The listing builds one solid part. Answer for the finished solid, in the listing's coordinates (mm). A direction names the side the tool comes from. Give positions to 0.01 mm unless a question says otherwise; leave off trailing zeros. Order: outer loops, then holes, each group sorted by start corner. A loop starts at its lowest first (then second) coordinate and runs counter-clockwise, first axis right, second up. Notation, with made-up numbers: (12.25, -39) - (62.25, -39) arc R19 cw to (62.25, -24) - close; hole circle Ø4 at (52, 39). An arc over 180 degrees is marked (long way). Write each question's results on one line, items separated by ' | '. Start each with the question number.
1. Find the intervals of material crossed by L1, parallel to X at y = -3.5, z = 14; L2, parallel to Z at x = 20, y = -3.25; L3, parallel to Y at x = 9, z = 0.5, in increasing order.
2. Section B-B (x = 31.5) is taken. Give the vertices of the cut face in (y, z), and give its area (3 significant figures).
3. Section C-C (z = -6.5) is taken. Give the vertices of the cut face in (x, y), and give its area (3 significant figures).
4. Section A-A (y = -3.75) is taken. Give the vertices of the cut face in (x, z).
5. A flat-ended cylindrical pin translates along its axis: pin 1 (15 mm diameter, centred on x = -17, z = 5, fed in from -Y). Find the tip coordinate at first contact, or state that the pin passes through.
6. Which of the six approach directions +Z, -Z, +X, -X, +Y, -Y give full straight-line access (tool end or side, diameter ignored) to faces 1 (the face through (53.85, -4, 0)), 2 (the face through (-1, 0, 0))?
7. Determine the mould class of faces 3 (the face through (-1, -3, -27.06)), 4 (the face through (-4.98, -4, 0)), 5 (the face through (-5, -6.65, 22)) for opening direction Z: released by +Z, released by -Z, zero draft, split by the parting line, or undercut.
from build123d import *

# Parameters (mm, degrees)
F0_W     = 121.7
F0_H     = 54.12
F1_DEPTH = 6.65
F2_W     = 27.26
F2_H     = 40.12
F2_W_2   = 18.61
F3_DEPTH = 4.85


with BuildPart() as f1:
    # F0 (on Front) → F1 (new body)
    with BuildSketch(Plane.XZ):
        Rectangle(F0_W, F0_H)
    extrude(amount=F1_DEPTH)

    # F2 (on face) → F3 (cut)
    with BuildSketch(Plane.XZ.offset(6.65)):
        with Locations((-40.22, 0)):
            Rectangle(F2_W, F2_H)
        with Locations((-15.785, 0)):
            Rectangle(F2_W_2, F2_H)
        with Locations((4.325, 0)):
            Rectangle(F2_W_2, F2_H)
        with Locations((24.435, 0)):
            Rectangle(F2_W_2, F2_H)
        with Locations((44.545, 0)):
            Rectangle(F2_W_2, F2_H)
    extrude(amount=-F3_DEPTH, mode=Mode.SUBTRACT)


solid = f1.part
Reported:
1) L1: -60.85 to -53.85, -26.59 to -25.09, -6.48 to -4.98, 13.63 to 15.13, 33.74 to 35.24, 53.85 to 60.85 | L2: -27.06 to -20.06, 20.06 to 27.06 | L3: -1.8 to 0
2) outline: (-6.65, -27.06) - (0, -27.06) - (0, 27.06) - (-6.65, 27.06) - (-6.65, 20.06) - (-1.8, 20.06) - (-1.8, -20.06) - (-6.65, -20.06) - close | area: 165 mm²
3) outline: (-60.85, -6.65) - (-53.85, -6.65) - (-53.85, -1.8) - (-26.59, -1.8) - (-26.59, -6.65) - (-25.09, -6.65) - (-25.09, -1.8) - (-6.48, -1.8) - (-6.48, -6.65) - (-4.98, -6.65) - (-4.98, -1.8) - (13.63, -1.8) - (13.63, -6.65) - (15.13, -6.65) - (15.13, -1.8) - (33.74, -1.8) - (33.74, -6.65) - (35.24, -6.65) - (35.24, -1.8) - (53.85, -1.8) - (53.85, -6.65) - (60.85, -6.65) - (60.85, 0) - (-60.85, 0) - close | area: 316 mm²
4) outline: (-60.85, -27.06) - (60.85, -27.06) - (60.85, 27.06) - (-60.85, 27.06) - close; hole (-53.85, -20.06) - (-26.59, -20.06) - (-26.59, 20.06) - (-53.85, 20.06) - close; hole (-25.09, -20.06) - (-6.48, -20.06) - (-6.48, 20.06) - (-25.09, 20.06) - close; hole (-4.98, -20.06) - (13.63, -20.06) - (13.63, 20.06) - (-4.98, 20.06) - close; hole (15.13, -20.06) - (33.74, -20.06) - (33.74, 20.06) - (15.13, 20.06) - close; hole (35.24, -20.06) - (53.85, -20.06) - (53.85, 20.06) - (35.24, 20.06) - close
5) pin 1: y = -1.8
6) face 1: -Y | face 2: +Z, -Z, +X, -X, +Y
7) face 3: released by -Z | face 4: undercut | face 5: zero draft
